from build123d import *

# Parameters (mm, degrees)
F1_DEPTH       = 82.55
F4_D           = 38.1
F4_CBORE_D     = 50.8
F4_CBORE_DEPTH = 12.7
F5_D           = 38.1
F5_CBORE_D     = 50.8
F5_CBORE_DEPTH = 12.7


with BuildPart() as f1:
    # F0 (on Front) → F1 (new body)
    with BuildSketch(Plane.XZ):
        with BuildLine():
            Line((0, 76.2), (0, 0))
            Line((0, 0), (177.8, 0))
            Line((177.8, 0), (177.8, 28.575))
            Line((177.8, 28.575), (82.55, 28.575))
            Line((82.55, 28.575), (82.55, 76.2))
            ThreePointArc((82.55, 76.2), (41.275, 117.475), (0, 76.2))
        make_face()
    extrude(amount=F1_DEPTH)

    # F4 (through all)
    with Locations(Plane.XZ.offset(82.55)):
        with Locations((41.275, 76.2)):
            CounterBoreHole(F4_D / 2, F4_CBORE_D / 2, F4_CBORE_DEPTH)

    # F5 (through all)
    with Locations(Plane.XY.offset(28.575)):
        with Locations((139.7, -39.375536)):
            CounterBoreHole(F5_D / 2, F5_CBORE_D / 2, F5_CBORE_DEPTH)


solid = f1.part
Geometry check sheet. Reference: the model listing, model coordinates, mm. A direction names the side the tool comes from. Give positions to 0.01 mm unless a question says otherwise; leave off trailing zeros. Order: outer loops, then holes, each group sorted by start corner. A loop starts at its lowest first (then second) coordinate and runs counter-clockwise, first axis right, second up. Notation, with made-up numbers: (1, 33) - (19, 33) arc R20 cw to (19, 67) - close; hole circle Ø5 at (-3, 53). An arc over 180 degrees is marked (long way). Answer as a JSON object with one key per item and string values.
(1) Cross-section at D-D (y = -72.5). Record the cut outline in (x, z) (3 decimals).
Report:
{"outline": "(0, 0) - (177.8, 0) - (177.8, 28.575) - (82.55, 28.575) - (82.55, 76.2) arc R41.275 ccw to (0, 76.2) - close; hole circle Ø50.8 at (41.275, 76.2)"}
(2) Cross-section at C-C (z = 60). Record the cut outline in (x, y), then the cut area to 3 significant figures.
Report:
{"outline": "(0, -82.55) - (21.71, -82.55) - (21.71, -69.85) - (31.25, -69.85) - (31.25, 0) - (0, 0) - close; (51.3, -69.85) - (60.84, -69.85) - (60.84, -82.55) - (82.55, -82.55) - (82.55, 0) - (51.3, 0) - close", "area": "4,920 mm^2"}
(3) Draft check along X on faces 1 (the cylindrical face through (42.183, -40.697, 117.465)), 2 (the flat face through (177.8, -41, 14)), 3 (the flat face through (68, 0, 47)), 4 (the cylindrical face through (31.03, -34.44, 92.26)). Enter one of: released by +X, released by -X, zero draft, split by the parting line, or undercut.
Report:
{"face 1": "split by the parting line", "face 2": "released by +X", "face 3": "zero draft", "face 4": "undercut"}
(4) Tool access check on faces 5 (the flat face through (88, -41, 0)), 6 (the cylindrical face through (163.163, -49.104, 22.314)), 7 (the flat face through (44.9, -69.85, 95.1)), 8 (the flat face through (110, -41, 28.575)), 9 (the cylindrical face through (158.73, -38.54, 7.83)). Record the directions out of +Z, -Z, +X, -X, +Y, -Y that give a thin tool (end or side, any length) a straight path to the whole face; none if there is none.
Report:
{"face 5": "-Z, +X, -X, +Y, -Y", "face 6": "+Z", "face 7": "-Y", "face 8": "+Z, +X, +Y, -Y", "face 9": "+Z, -Z"}
(5) Material ranges on line 1 (X direction, y = -55, z = 76); line 2 (Z direction, x = 147, y = -57) (3 decimals); line 3 (Y direction, x = 139, z = 21), recorded low to high.
Report:
{"line 1": "0 to 22.23, 60.32 to 82.55", "line 2": "0 to 15.875", "line 3": "-82.55 to -64.77, -13.99 to 0"}
(6) Depth check by flat-ended pin: pin 1 Ø1 at (x, y) = (89.5, -51.5) entering from +Z (3 decimals); pin 2 Ø12 at (y, z) = (-38.5, 31) entering from +X; pin 3 Ø1.5 at (x, y) = (78.5, -66.5) entering from +Z; pin 4 Ø8 at (x, y) = (78, -37.5) entering from +Z. Enter the tip coordinate at first touch or a pass-through.
Report:
{"pin 1": "z = 28.575", "pin 2": "x = 177.8", "pin 3": "z = 95.52", "pin 4": "z = 101.35"}
(7) Cross-section at A-A (x = 139.7). Record the cut outline in (y, z) (3 decimals).
Report:
{"outline": "(-82.55, 0) - (-58.426, 0) - (-58.426, 15.875) - (-64.776, 15.875) - (-64.776, 28.575) - (-82.55, 28.575) - close; (-20.326, 0) - (0, 0) - (0, 28.575) - (-13.976, 28.575) - (-13.976, 15.875) - (-20.326, 15.875) - close"}
(8) Cross-section at B-B (y = -30.5). Record the cut outline in (x, z) (3 decimals), then the cut area to 3 significant figures.
Report:
{"outline": "(0, 0) - (122.844, 0) - (122.844, 15.875) - (115.901, 15.875) - (115.901, 28.575) - (82.55, 28.575) - (82.55, 76.2) arc R41.275 ccw to (0, 76.2) - close; (156.556, 0) - (177.8, 0) - (177.8, 28.575) - (163.499, 28.575) - (163.499, 15.875) - (156.556, 15.875) - close; hole circle Ø38.1 at (41.275, 76.2)", "area": "9,410 mm^2"}
